Read the model definition and answer for the solid it produces. Units are mm, in the model's axes. A direction names the side the tool comes from. Coordinates: 2 decimals unless noted, no trailing zeros. Write each loop counter-clockwise with the first axis right and the second up, starting at its lowest first coordinate (ties: lowest second). Pieces come first, ordered by that corner, then holes. Notation, with made-up numbers: (28, 10) -> (72, 10) arc R15 ccw to (72, 15) -> close; hole circle Ø1 at (73, 67). An arc over 180 degrees is marked (long way). Answer as a JSON object with one key per item and string values. Group by question number.
(1) Find section A-A (z = -35). Give the vertices of the cut face in (x, y), then the cut area to 3 significant figures.
(2) Which of the six approach directions +Z, -Z, +X, -X, +Y, -Y give full straight-line access (tool end or side, diameter ignored) to faces 4 (the face through (30, -11, -63)), 5 (the face through (52.31, -9.7, -3.85)), 6 (the face through (30, -9, 0))?
(3) Flat-ended cylindrical pins translate along their axes: P1, Ø6, axis at y = -4, z = -19, coming from the +X side; P2, Ø4, axis at x = 47.5, z = -33.5, coming from the -Y side; P3, Ø2.5, axis at x = 53.65, z = -3.68, coming from the -Y side. Find the tip coordinate at first contact, or state that the pin passes through.
(4) Find section D-D (y = -20.25). Give the vertices of the cut face in (x, z).
(5) Find section B-B (x = 45.5). Give the vertices of the cut face in (y, z) (1 decimal).
(6) Straight lines are drawn through the part: L1, parallel to X at y = 1.55, z = -42; L2, parallel to Z at x = 20.5, y = -14; L3, parallel to X at y = -6.5, z = -67. For each, find the intervals that lie inside material, in ascending order.
(7) Find section C-C (z = -42). Give the vertices of the cut face in (x, y).
(8) For a pull along Z with two mould halves and no side action, classify faces 1 (the face through (30, -9, -70)), 2 (the face through (60, 1, -32)), 3 (the face through (46.01, 2.33, -40.39)) as +Z half, -Z half, draft (parallel to the pull), parting line (faces both ways), or undercut.
from build123d import *

# Parameters (mm, degrees)
SKETCH2_W                      = 60
SKETCH2_H                      = 70
BOSS_EXTRUDE1_DEPTH            = 4.5974
SKETCH4_R                      = 6.1905
SKETCH4_R_2                    = 1.6905
CUT_EXTRUDE1_DEPTH             = 93.309999928
SKETCH5_W                      = 60
SKETCH5_H                      = 22.225
BOSS_EXTRUDE2_DEPTH            = 7
F_6_32_TAPPED_HOLE1_AT_2_COUNT = 2
F_6_32_TAPPED_HOLE1_AT_2_PITCH = 47.298975859


with BuildPart() as part:
    # Sketch2 → Boss-Extrude1 (new body)
    with BuildSketch(Plane(origin=(0, 0, 0), x_dir=(1, 0, 0), z_dir=(0, 1, 0))):
        with Locations((30, 35)):
            Rectangle(SKETCH2_W, SKETCH2_H)
    extrude(amount=BOSS_EXTRUDE1_DEPTH)

    # Sketch4 → Cut-Extrude1 (cut, through all)
    with BuildSketch(Plane(origin=(0, 4.5974, 0), x_dir=(1, 0, 0), z_dir=(0, 1, 0))):
        with Locations(Location((30, 35, 0), (0, 0, 270))):
            Circle(SKETCH4_R)
        with Locations(Location((45.5, 42, 0), (0, 0, 270))):
            Circle(SKETCH4_R_2)
        with Locations(Location((14.5, 42, 0), (0, 0, 270))):
            Circle(SKETCH4_R_2)
    extrude(amount=-CUT_EXTRUDE1_DEPTH, mode=Mode.SUBTRACT)

    # Sketch5 → Boss-Extrude2 (add)
    with BuildSketch(Plane(origin=(0, 0, -70), x_dir=(-1, 0, 0), z_dir=(0, 0, -1))):
        with Locations((-30, -11.1125)):
            Rectangle(SKETCH5_W, SKETCH5_H)
    boss_extrude2 = extrude(amount=-BOSS_EXTRUDE2_DEPTH)

    # Sketch8 → #6-32 Tapped Hole1 (revolve, cut)
    with BuildSketch(Plane(origin=(6.35104386, -22.225, -66.368109228), x_dir=(0, 0, -1), z_dir=(1, 0, 0))):
        Polygon((0, 0), (0, 26.21269403), (1.35255, 25.4), (1.35255, 0), align=None)
    f_6_32_tapped_hole1 = revolve(axis=Axis((6.35104386, -28.575, -66.368109228), (0, 1, 0)), mode=Mode.SUBTRACT)

    # #6-32 Tapped Hole1 at 2: #6-32 Tapped Hole1 ×2
    with Locations(*[Vector(0.9999995830982151, 0, 0.0009131283567521887) * (i * F_6_32_TAPPED_HOLE1_AT_2_PITCH) for i in range(1, F_6_32_TAPPED_HOLE1_AT_2_COUNT)]):
        add(f_6_32_tapped_hole1, mode=Mode.SUBTRACT)

    # Mirror1: Boss-Extrude2, #6-32 Tapped Hole1 across plane
    add(boss_extrude2.mirror(Plane(origin=(0, 0, -35), x_dir=(1, 0, 0), z_dir=(0, 0, -1))))
    add(f_6_32_tapped_hole1.mirror(Plane(origin=(0, 0, -35), x_dir=(1, 0, 0), z_dir=(0, 0, -1))), mode=Mode.SUBTRACT)

    # Mirror1 copy 1 sketch → Mirror1 copy 1 (revolve, cut)
    with BuildSketch(Plane(origin=(53.65, -22.225, -3.675080808), x_dir=(0, 0, 1), z_dir=(1, 0, 0))):
        Polygon((0, 0), (0, -26.21269403), (1.35255, -25.4), (1.35255, 0), align=None)
    revolve(axis=Axis((53.65, -28.575, -3.675080808), (0, -1, 0)), mode=Mode.SUBTRACT)


solid = part.part
Results below:
{
 "1": {"outline": "(0, 0) -> (23.81, 0) -> (23.81, 4.6) -> (0, 4.6) -> close; (36.19, 0) -> (60, 0) -> (60, 4.6) -> (36.19, 4.6) -> close", "area": "219 mm2"},
 "2": {"face 4": "+X, -X, -Y", "face 5": "-Y", "face 6": "+Z, +X, -X, +Y, -Y"},
 "3": {"P1": "passes through", "P2": "stops at y = 0", "P3": "stops at y = 3.23"},
 "4": {"outline": "(0, -70) -> (60, -70) -> (60, -63) -> (0, -63) -> close; (0, -7) -> (60, -7) -> (60, 0) -> (0, 0) -> close; hole circle Ø2.71 at (6.35, -66.37); hole circle Ø2.71 at (6.35, -3.63); hole circle Ø2.71 at (53.65, -66.32); hole circle Ø2.71 at (53.65, -3.68)"},
 "5": {"outline": "(-22.2, -70) -> (4.6, -70) -> (4.6, -43.7) -> (0, -43.7) -> (0, -63) -> (-22.2, -63) -> close; (-22.2, -7) -> (0, -7) -> (0, -40.3) -> (4.6, -40.3) -> (4.6, 0) -> (-22.2, 0) -> close"},
 "6": {"L1": "x = 0 to 12.81, 16.19 to 43.81, 47.19 to 60", "L2": "z = -70 to -63, -7 to 0", "L3": "x = 0 to 5.16, 7.55 to 52.48, 54.82 to 60"},
 "7": {"outline": "(0, 0) -> (12.81, 0) -> (12.81, 4.6) -> (0, 4.6) -> close; (16.19, 0) -> (43.81, 0) -> (43.81, 4.6) -> (16.19, 4.6) -> close; (47.19, 0) -> (60, 0) -> (60, 4.6) -> (47.19, 4.6) -> close"},
 "8": {"face 1": "-Z half", "face 2": "draft", "face 3": "undercut"}
}
